Work out the finished part from the listing and answer in its coordinate system (mm). Face numbers are marked on the shaded views. Give positions to 0.01 mm unless a question says otherwise; leave off trailing zeros. Loops run counter-clockwise (first coordinate to the right, second up) from the corner with the lowest first, then second, coordinate; pieces in that order, holes last. Notation, with made-up numbers: M 44,-11 L 52,-11 A11 cw 52,10 Z; hole C -12,-35 d11. An arc over 180 degrees is marked long. Answer as a JSON object with one key per item and string values. Group by question number.
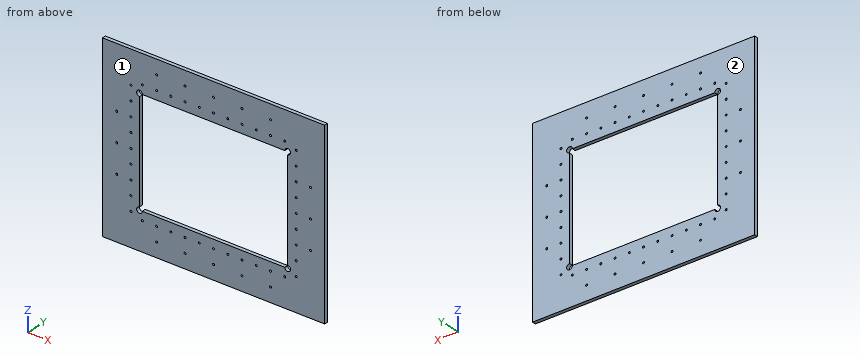
```python
from build123d import *

# Parameters (mm, degrees)
F0_W     = 780
F0_H     = 630
F0_W_2   = 520
F0_H_2   = 370
F1_DEPTH = 12.7
F4_D     = 6.7056
F5_R     = 10
F6_DEPTH = 12.701


with BuildPart() as f1:
    # F0 (on Front) → F1 (new body)
    with BuildSketch(Plane.XZ):
        Rectangle(F0_W, F0_H)
        Rectangle(F0_W_2, F0_H_2, mode=Mode.SUBTRACT)
    extrude(amount=-F1_DEPTH)

    # F4 (through all)
    with Locations(Plane.XZ):
        with Locations((-250, 215), (-200, 215), (-150, 215), (-100, 215), (-50, 215), (0, 215), (50, 215), (100, 215), (150, 215), (200, 215), (250, 215), (200, 265), (100, 265), (0, 265), (-100, 265), (-200, 265), (-290, 200), (-290, 150), (-290, 100), (-290, 50), (-290, 0), (-340, 0), (-340, 100), (-290, -50), (-290, -100), (-290, -150), (100, -265), (0, -265), (200, -265), (-100, -265), (-200, -265), (100, -215), (-100, -215), (-200, -215), (250, -215), (150, -215), (-50, -215), (-150, -215), (0, -215), (50, -215), (-250, -215), (200, -215), (-290, -200), (290, 50), (290, 0), (290, 200), (290, 150), (290, 100), (290, -200), (290, -150), (290, -100), (290, -50), (-340, -100), (340, 100), (340, 0), (340, -100), (340, 0), (340, -100)):
            Hole(F4_D / 2)

    # F5 (on face) → F6 (cut, through all)
    with BuildSketch(Plane.XZ):
        with Locations((-260, 185)):
            Circle(F5_R)
        with Locations((-260, -185)):
            Circle(F5_R)
        with Locations((260, -185)):
            Circle(F5_R)
        with Locations((260, 185)):
            Circle(F5_R)
    extrude(amount=-F6_DEPTH, mode=Mode.SUBTRACT)


solid = f1.part
```
Item 1: Given pin 1 Ø6 at (x, z) = (-150, 215) entering from +Y, flat-ended and moving along its own axis, determine where the tip first touches the part or whether it passes through.
Item 2: A cutting plane is placed at B-B (z = -136). Determine the outline of the cut face in (x, y).
Item 3: Find the intervals of material crossed by probe 1 along Z at (x, y) = (0, 4.75); probe 2 along Z at (x, y) = (150, 7.5); probe 3 along Z at (x, y) = (340, 3.5), in increasing order. Write a range as [from, to].
Item 4: A cutting plane is placed at C-C (y = 5.25). Give the number of separate pieces and of enclosed holes in the cut face, and give its area (3 significant figures).
Item 5: For a pull along Y with two mould halves and no side action, classify the marked faces 1 and 2 as pulls with the +Y half, pulls with the -Y half, needs draft (parallel to the pull), parting line crosses it, or undercut.
Item 6: A cutting plane is placed at A-A (x = -218.5). Determine the outline of the cut face in (y, z), and give its area (3 significant figures).
The answers:
{
 "1": {"pin 1": "passes through"},
 "2": {"outline": "M -390,0 L -260,0 L -260,12.7 L -390,12.7 Z; M 260,0 L 390,0 L 390,12.7 L 260,12.7 Z"},
 "3": {"probe 1": "z = [-315, -268.35], [-261.65, -218.35], [-211.65, -185], [185, 211.65], [218.35, 261.65], [268.35, 315]", "probe 2": "z = [-315, -218.35], [-211.65, -185], [185, 211.65], [218.35, 315]", "probe 3": "z = [-315, -103.35], [-96.65, -3.35], [3.35, 96.65], [103.35, 315]"},
 "4": {"separate pieces": "1", "enclosed holes": "57", "area": "296,000 mm^2"},
 "5": {"face 1": "pulls with the -Y half", "face 2": "pulls with the +Y half"},
 "6": {"outline": "M 0,-315 L 12.7,-315 L 12.7,-185 L 0,-185 Z; M 0,185 L 12.7,185 L 12.7,315 L 0,315 Z", "area": "3,300 mm^2"}
}
